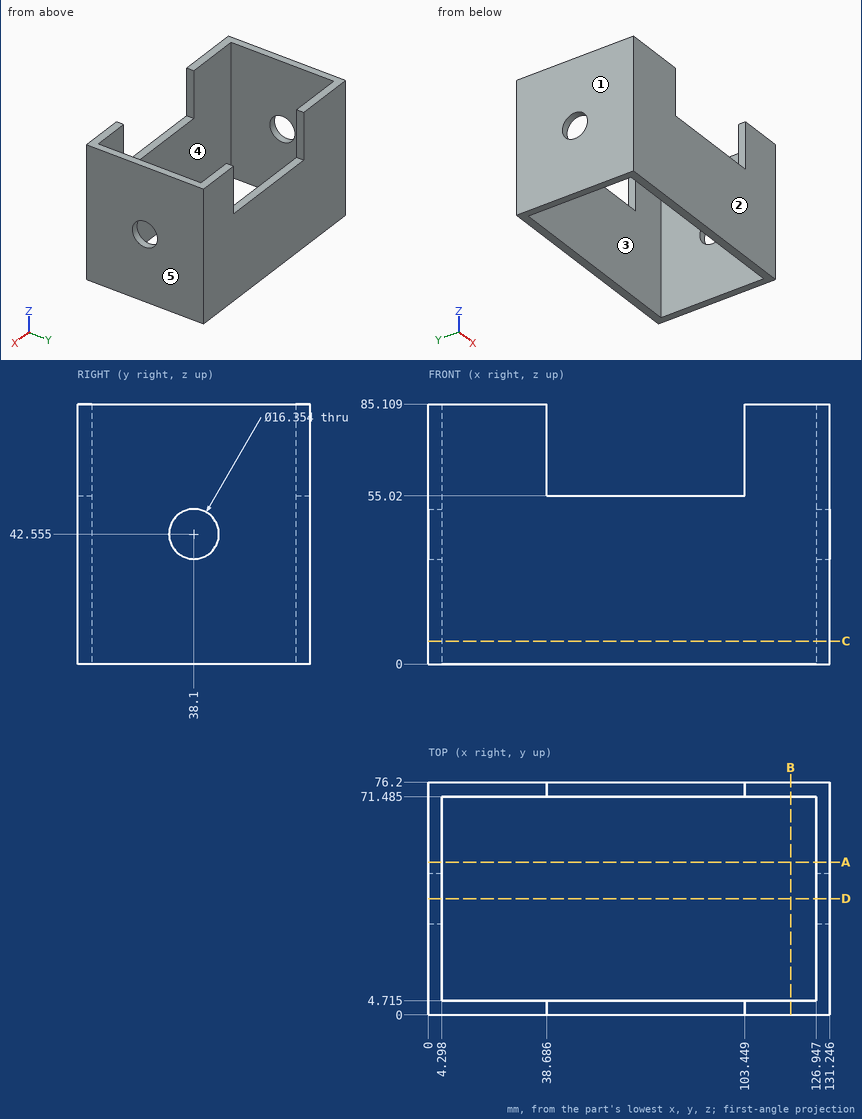
Study the drawing (mm; zero at the part's minimum x, y, z) and answer. A direction names the side the tool comes from. Give positions to 0.01 mm unless a question says otherwise; leave off trailing zeros. Order: outer loops, then holes, each group sorted by start corner. A loop starts at its lowest first (then second) coordinate and runs counter-clockwise, first axis right, second up.
1) Find section D-D on y = 38.1. Write down the section's boundary in (x, z) (1 decimal), then the cut area to 3 significant figures.
Reported:
outline: (0, 0) - (4.3, 0) - (4.3, 34.4) - (0, 34.4) - close; (0, 50.7) - (4.3, 50.7) - (4.3, 85.1) - (0, 85.1) - close; (126.9, 0) - (131.2, 0) - (131.2, 34.4) - (126.9, 34.4) - close; (126.9, 50.7) - (131.2, 50.7) - (131.2, 85.1) - (126.9, 85.1) - close
area: 591 mm2
2) Consider line 1 along X through (y, z) = (5, 19.5) (1 decimal); line 2 along Y through (x, z) = (58.5, 48.5) (1 decimal); line 3 along Z through (x, y) = (1.3, 38.1). Determine where each line is inside the solid, lowest interval first.
Reported:
line 1: x = 0 to 4.3, 126.9 to 131.2
line 2: y = 0 to 4.7, 71.5 to 76.2
line 3: z = 0 to 34.38, 50.73 to 85.11
3) Find section A-A on y = 50. Write down the section's boundary in (x, z) (1 decimal).
Reported:
outline: (0, 0) - (4.3, 0) - (4.3, 85.1) - (0, 85.1) - close; (126.9, 0) - (131.2, 0) - (131.2, 85.1) - (126.9, 85.1) - close
4) For the marked faces 4 and 5, determine the directions among +Z, -Z, +X, -X, +Y, -Y from which every point of the face is accessible in a straight line to the end or side of a thin tool.
Reported:
face 4: +Z, -Z
face 5: +Z, -Z, +X, +Y, -Y
5) Find section C-C on z = 7.5. Write down the section's boundary in (x, y) (1 decimal).
Reported:
outline: (0, 0) - (131.2, 0) - (131.2, 76.2) - (0, 76.2) - close; hole (4.3, 4.7) - (126.9, 4.7) - (126.9, 71.5) - (4.3, 71.5) - close
6) Find section B-B on x = 118.5. Write down the section's boundary in (y, z) (1 decimal).
Reported:
outline: (0, 0) - (4.7, 0) - (4.7, 85.1) - (0, 85.1) - close; (71.5, 0) - (76.2, 0) - (76.2, 85.1) - (71.5, 85.1) - close
7) Given P1, Ø6, axis at y = 23.5, z = 55, coming from the -X side; P2, Ø1.4, axis at x = 71.5, y = 2, coming from the +Z side; P3, Ø13, axis at y = 38.1, z = 42.55, coming from the -X side, each flat-ended and moving along its own axis, determine where each tip first touches the part or whether it passes through.
Reported:
P1: stops at x = 0
P2: stops at z = 55.02
P3: passes through
8) Determine the mould class of the marked faces 1, 2 and 3 for opening direction X: pulls with the +X half, pulls with the -X half, needs draft (parallel to the pull), parting line crosses it, or undercut.
Reported:
face 1: pulls with the -X half
face 2: needs draft
face 3: undercut
